Autodesk Inventor part; units mm, degrees
ref_plane "YZ Plane" through (0, 0, 0) normal (1, 0, 0) x (0, 1, 0)
ref_plane "XZ Plane" through (0, 0, 0) normal (0, 1, 0) x (-1, 0, 0)
ref_plane "XY Plane" through (0, 0, 0) normal (0, 0, 1) x (1, 0, 0)
sketch "Sketch1" plane through (0, 0, 0) normal (0, 1, 0) x (-1, 0, 0)
  circle A0 centre (0, 0) radius 6.5
  circle A1 centre (0, 0) radius 7.5
  dimension "d0" = 13
  dimension "d1" = 15
extrude "Extrusion1" add sketch "Sketch1" along normal blind 10
sketch "Sketch2" plane through (0, 10, 0) normal (0, 1, 0) x (1, 0, 0)
  line L0 (-93.2796, -95.8103) -> (93.2796, 95.8103) construction
  line L1 (93.2796, -95.8103) -> (-93.2796, 95.8103) construction
  circle A0 centre (0, 0) radius 7.5
  line L2 (-7.5, 0) -> (-93.2796, 95.8103)
  line L3 (-93.2796, 95.8103) -> (0, 7.5)
  line L4 (0, 7.5) -> (93.2796, 95.8103)
  line L5 (93.2796, 95.8103) -> (7.5, 0)
  line L6 (7.5, 0) -> (93.2796, -95.8103)
  line L7 (93.2796, -95.8103) -> (0, -7.5)
  line L8 (0, -7.5) -> (-93.2796, -95.8103)
  line L9 (-93.2796, -95.8103) -> (-7.5, 0)
extrude "Extrusion2" add sketch "Sketch2" along normal blind 10
sketch "Sketch3" plane through (0, 10, 0) normal (0, -1, 0) x (1, 0, 0)
  point P0 (0, 0)
sketch "Sketch4" plane through (0, 20, 0) normal (0, 1, 0) x (1, 0, 0)
  circle A0 centre (0, 0) radius 6.5
extrude "Extrusion3" cut sketch "Sketch4" against normal through all
properties part number "Ventilador Pieza extra de ensamble SEBASTIAN BERMUDEZ"
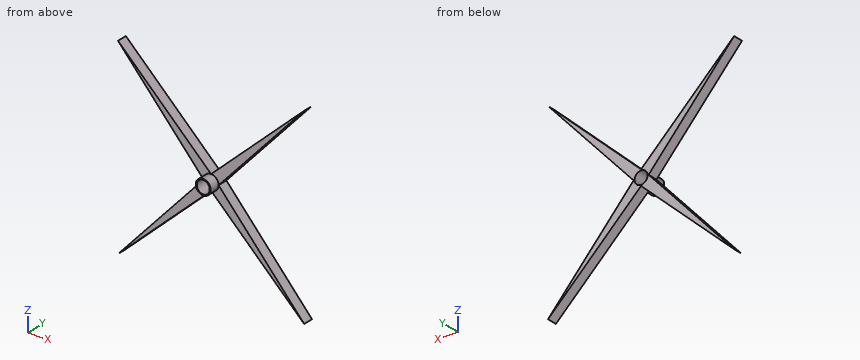
CAD build for the part. Positions are in the model's coordinates, mm. Round coordinates to 2 decimals unless told otherwise and drop trailing zeros. Write each loop counter-clockwise with the first axis right and the second up, starting at its lowest first coordinate (ties: lowest second). Pieces come first, ordered by that corner, then holes.
Item 1: Band-saw the part on A-A on y = 13.5. Write the cut outline in (x, z), then the cut area to 3 significant figures.
Filled in:
outline: (-93.28, -95.81) - (0, -7.5) - (93.28, -95.81) - (7.5, 0) - (93.28, 95.81) - (0, 7.5) - (-93.28, 95.81) - (-7.5, 0) - close; hole circle Ø13 at (0, 0)
area: 2,700 mm2
Item 2: Band-saw the part on B-B on x = -35. Write the cut outline in (y, z), then the cut area to 3 significant figures.
Filled in:
outline: (10, -40.64) - (20, -40.64) - (20, -30.72) - (10, -30.72) - close; (10, 30.72) - (20, 30.72) - (20, 40.64) - (10, 40.64) - close
area: 198 mm2
Item 3: Band-saw the part on C-C on z = -27. Write the cut outline in (x, y).
Filled in:
outline: (-31.67, 10) - (-20.6, 10) - (-20.6, 20) - (-31.67, 20) - close; (20.6, 10) - (31.67, 10) - (31.67, 20) - (20.6, 20) - close
Item 4: Drill centre lines: L1, parallel to X at y = 9, z = 0; L2, parallel to X at y = 17.5, z = -10.5. Where is each one in solid material? Low to high.
Filled in:
L1: x = -7.5 to -6.5, 6.5 to 7.5
L2: x = -16.9 to -3.17, 3.17 to 16.9
Item 5: Drop flat-ended pins along their axis: pin 1 Ø5 at (y, z) = (9, -65.5) entering from -X; pin 2 Ø10 at (x, y) = (-6, 6.5) entering from -Z; pin 3 Ø4 at (y, z) = (16, 26.5) entering from -X. Give the stop position or say it passes through.
Filled in:
pin 1: stops at x = -68.19
pin 2: stops at z = -16.56
pin 3: stops at x = -33.02
